```python
from build123d import *

# Parameters (mm, degrees)
F2_W     = 1500
F2_H     = 1500
F0_DEPTH = 1500
F1_R     = 100
F3_W     = 1300
F3_H     = 1300
F3_W_2   = 284
F3_H_2   = 284
F4_DEPTH = 1500


with BuildPart() as f0:
    # F2 (on Top) → F0 (new body)
    with BuildSketch(Plane.XY):
        Rectangle(F2_W, F2_H)
    extrude(amount=F0_DEPTH)

    # F1
    f1_edges = [f0.edges().sort_by_distance(p)[0] for p in [
        (0, -750, 1500),
        (750, 0, 1500),
        (0, 750, 1500),
        (-750, 0, 1500),
    ]]
    fillet(f1_edges, radius=F1_R)

    # F3 (on face) → F4 (cut)
    with BuildSketch(Plane.XY.offset(1500)):
        Rectangle(F3_W, F3_H)
        Rectangle(F3_W_2, F3_H_2, mode=Mode.SUBTRACT)
        Rectangle(F3_W_2, F3_H_2)
    extrude(amount=-F4_DEPTH, mode=Mode.SUBTRACT)


solid = f0.part
```
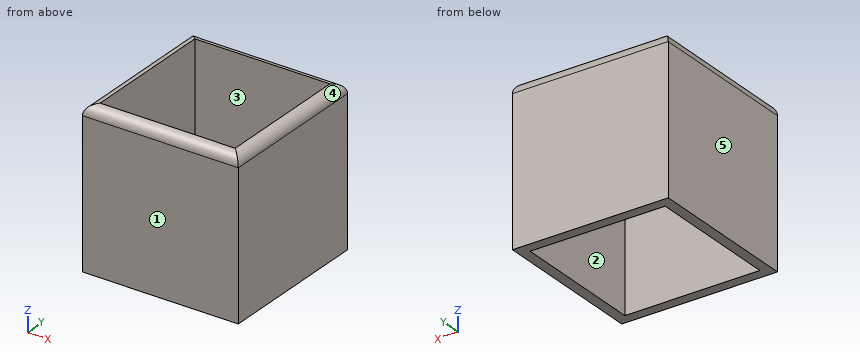
Can you work these out from the model? Positions are in its coordinate system, mm. Face numbers are marked on the shaded views. A direction names the side the tool comes from. Round coordinates to 2 decimals unless told otherwise and drop trailing zeros. Loops run counter-clockwise (first coordinate to the right, second up) from the corner with the lowest first, then second, coordinate; pieces in that order, holes last.
Item 1: If we mould it in two halves opening along X, with no side actions, what happens to the marked faces 3, 4 and 5? For each: +X half, -X half, draft (parallel to the pull), parting line (faces both ways), or undercut.
Item 2: Suppose I cut it at C-C, the plane z = 638.5. Write out the boundary of the cut face in (x, y).
Item 3: Which directions (+Z, -Z, +X, -X, +Y, -Y) give clear straight access to the entire face, cutting with the end or side of a thin tool? Please do the marked faces 1 and 2.
Item 4: Suppose I cut it at A-A, the plane y = -568.5. Write out the boundary of the cut face in (x, z).
Item 5: Please list where these lines run through material, in increasing order: L1, parallel to X at y = -633, z = 1297; L2, parallel to Y at x = -319, z = 1406.5.
Reported:
1. face 3: undercut
1. face 4: +X half
1. face 5: -X half
2. outline: (-750, -750) - (750, -750) - (750, 750) - (-750, 750) - close; hole (-650, -650) - (650, -650) - (650, 650) - (-650, 650) - close
3. face 1: +Z, -Z, +X, -X, -Y
3. face 2: +Z, -Z
4. outline: (-750, 0) - (-650, 0) - (-650, 1500) arc R100 ccw to (-750, 1400) - close; (650, 0) - (750, 0) - (750, 1400) arc R100 ccw to (650, 1500) - close
5. L1: x = -750 to -650, 650 to 750
5. L2: y = -749.79 to -650, 650 to 749.79
